```python
from build123d import *

# Parameters (mm, degrees)
ESQUISSE1_W             = 30
ESQUISSE1_H             = 10
ESQUISSE4_R             = 1.5
ESQUISSE4_W             = 3
ESQUISSE4_H             = 2.501285573
ESQUISSE5_W             = 24.738109029
ESQUISSE5_H             = 14.721675616
ENL_V_MAT_EXTRU_2_DEPTH = 34.166247904


with BuildPart() as part:
    # Esquisse1 → Révolution2 (revolve)
    with BuildSketch(Plane.XY, mode=Mode.PRIVATE) as r_volution2_sk:
        with Locations((15, 5)):
            Rectangle(ESQUISSE1_W, ESQUISSE1_H)
    revolve(r_volution2_sk.sketch.rotate(Axis((0, 0, 0), (1, 0, 0)), 90), axis=Axis((0, 0, 0), (1, 0, 0)))

    # Esquisse4 → Enlèvement de matière-Révolution1 (revolve, cut)
    with BuildSketch(Plane(origin=(0, 0, 0), x_dir=(1, 0, 0), z_dir=(0, 1, 0)), mode=Mode.PRIVATE) as enl_vement_de_mati_re_r_volution1_sk:
        with Locations((11.370683678, 10)):
            Circle(ESQUISSE4_R)
        with Locations((21.404481516, 9.750642787)):
            Rectangle(ESQUISSE4_W, ESQUISSE4_H)
    revolve(enl_vement_de_mati_re_r_volution1_sk.sketch.rotate(Axis((0, 0, 0), (1, 0, 0)), 180), axis=Axis((0, 0, 0), (1, 0, 0)), mode=Mode.SUBTRACT)

    # Esquisse5 → Enlèv. mat.-Extru.2 (cut, through all)
    with BuildSketch(Plane(origin=(30, 0, 0), x_dir=(0, 0, -1), z_dir=(1, 0, 0))):
        with Locations((-12.369054515, -7.360837808)):
            Rectangle(ESQUISSE5_W, ESQUISSE5_H)
    extrude(amount=-ENL_V_MAT_EXTRU_2_DEPTH, mode=Mode.SUBTRACT)


solid = part.part
```
The model under review builds one solid part; all positions refer to its coordinate system, in mm. A direction names the side the tool comes from. Round coordinates to 2 decimals unless told otherwise and drop trailing zeros. Loops run counter-clockwise (first coordinate to the right, second up) from the corner with the lowest first, then second, coordinate; pieces in that order, holes last. Notation, with made-up numbers: M -24.75,34.5 L 7.25,34.5 A21 ccw 7.25,44.5 Z; hole C 19.25,56 d4. An arc over 180 degrees is marked long. Put each result on its own line as item: value.
Q1. Consider section A-A, the plane x = 24. Give the boundary of the cut face in (y, z).
Result set:
outline: M -10,0 A10 ccw long 0,10 L 0,0 Z
Q2. For pin 1 (2 mm diameter, centred on x = 3, y = -5.5, fed in from -Z); pin 2 (8 mm diameter, centred on x = 11, z = -6.5, fed in from -Y); pin 3 (3 mm diameter, centred on x = 12.5, y = -1, fed in from -Z); pin 4 (4 mm diameter, centred on x = 25, y = -7.5, fed in from -Z), all flat-tipped, find the tip position at first contact; note any pin that passes through.
Result set:
pin 1: stops at z = -8.93
pin 2: stops at y = -9.64
pin 3: stops at z = -10
pin 4: stops at z = -8.35
Q3. Mouldability with a two-part tool opening along X and no side actions: class faces 4 (the flat face through (0, 2, -2)), 5 (the cylindrical face through (21.425, 5.809, -6.205)), 6 (the cylindrical face through (26.502, 6.834, -7.3)), 7 (the flat face through (30, 2, -2)) as released by +X, released by -X, zero draft, split by the parting line, or undercut.
Result set:
face 4: released by -X
face 5: undercut
face 6: zero draft
face 7: released by +X
Q4. Machinability: for faces 1 (the flat face through (19.904, 7, -6)), 2 (the cylindrical face through (5.004, 6.834, -7.3)), 3 (the flat face through (15, 0, 5)), which of the approach directions +Z, -Z, +X, -X, +Y, -Y give a long, thin tool a straight path to every point of the face, cutting with its end or side? Answer none if there is none.
Result set:
face 1: none
face 2: +X, -X
face 3: +Z, +X, -X, -Y
Q5. To check wall thickness, follow L1, parallel to X at y = -7.5, z = -6.5; L2, parallel to X at y = 3, z = 9; L3, parallel to Z at x = 15, y = -0.25. State the ranges of each line that lie inside material, in increasing order.
Result set:
L1: x = 0 to 9.87, 12.87 to 19.9, 22.9 to 30
L2: x = 0 to 9.96, 12.78 to 19.9, 22.9 to 30
L3: z = -10 to 0
